from build123d import *

# Parameters (mm, degrees)
F2_R = 5.08
F3_R = 1.27


with BuildPart() as f1:
    # F0 (on Front) → F1 (revolve)
    with BuildSketch(Plane.XZ):
        with BuildLine():
            Line((-15.494, 0), (-8.636, 0))
            Line((-8.636, 0), (-8.636, 6.604))
            Line((-8.636, 6.604), (-5.1435, 10.0965))
            Line((-5.1435, 10.0965), (-5.1435, 32.004))
            Line((-5.1435, 32.004), (0, 37.1475))
            Line((0, 37.1475), (0, 53.4924))
            ThreePointArc((0, 53.4924), (-5.425442, 54.47622), (-10.16, 57.3024))
            Line((-10.16, 57.3024), (-13.335, 57.3024))
            Line((-13.335, 57.3024), (-13.335, 47.7774))
            Line((-13.335, 47.7774), (-7.9375, 45.812871))
            ThreePointArc((-7.9375, 45.812871), (-10.215656, 24.228081), (-15.494, 3.175))
            Line((-15.494, 3.175), (-15.494, 0))
        make_face()
    revolve(axis=Axis((0, 0, 48.82799), (0, 0, 1)))

    # F2
    f2_edges = [f1.edges().sort_by_distance(p)[0] for p in [
        (7.9375, 0, 45.812871),
    ]]
    fillet(f2_edges, radius=F2_R)

    # F3
    f3_edges = [f1.edges().sort_by_distance(p)[0] for p in [
        (13.335, 0, 47.7774),
        (13.335, 0, 57.3024),
    ]]
    fillet(f3_edges, radius=F3_R)


solid = f1.part
Work out the finished part from the listing and answer in its coordinate system (mm). A direction names the side the tool comes from. Round coordinates to 2 decimals unless told otherwise and drop trailing zeros. Write each loop counter-clockwise with the first axis right and the second up, starting at its lowest first coordinate (ties: lowest second). Pieces come first, ordered by that corner, then holes.
1) Straight lines are drawn through the part: line 1 (Y direction, x = 0, z = 2.75); line 2 (X direction, y = 0, z = 19). For each, find the intervals that lie inside material, in ascending order.
2) A cutting plane is placed at C-C (z = 38.5). Give the vertices of the cut face in (x, y).
3) Given pin 1 Ø4 at (x, z) = (-0.5, 50.5) entering from -Y (3 decimals); pin 2 Ø2 at (y, z) = (4.5, 29.5) entering from +X; pin 3 Ø10 at (y, z) = (10.5, 35.5) entering from -X; pin 4 Ø1.5 at (x, z) = (-12, 22.5) entering from -Y, each flat-ended and moving along its own axis, determine where each tip first touches the part or whether it passes through.
4) A cutting plane is placed at A-A (z = 52.5). Give the vertices of the cut face in (x, y) (3 decimals).
5) A tool of negligible diameter and unlimited length cuts with its end or side. For faces 1 (the cylindrical face through (1.74, -13.22, 52.3)), 2 (the flat face through (-7, 7, 0)), 3 (the cylindrical face through (1.124, -8.563, 3.348)), from which of +Z, -Z, +X, -X, +Y, -Y can it reach the whole face along a straight path? Write none if from no direction.
6) A cutting plane is placed at B-B (z = 18.5). Give the vertices of the cut face in (x, y), plus the area to 3 significant figures.
Completed:
1. line 1: y = -15.49 to -8.64, 8.64 to 15.49
1. line 2: x = -11.24 to -5.14, 5.14 to 11.24
2. outline: circle Ø16.73 at (0, 0)
3. pin 1: stops at y = -13.335
3. pin 2: stops at x = 8.73
3. pin 3: stops at x = -6.72
3. pin 4: passes through
4. outline: circle Ø26.67 at (0, 0)
5. face 1: +Z
5. face 2: -Z, +X, -X, +Y, -Y
5. face 3: -Z
6. outline: circle Ø22.69 at (0, 0); hole circle Ø10.29 at (0, 0)
6. area: 321 mm2
